For this review, use the dimensioned drawing (mm, ordinates from the lowest corner) and the shaded views. Coordinates: 2 decimals unless noted, no trailing zeros. Loops run counter-clockwise (first coordinate to the right, second up) from the corner with the lowest first, then second, coordinate; pieces in that order, holes last. Notation, with made-up numbers: (27, 19.5) -> (70, 19.5) arc R25 cw to (70, 31.5) -> close; hole circle Ø9 at (-3.5, 71). An arc over 180 degrees is marked (long way). Answer as a JSON object with one key per item and string values.
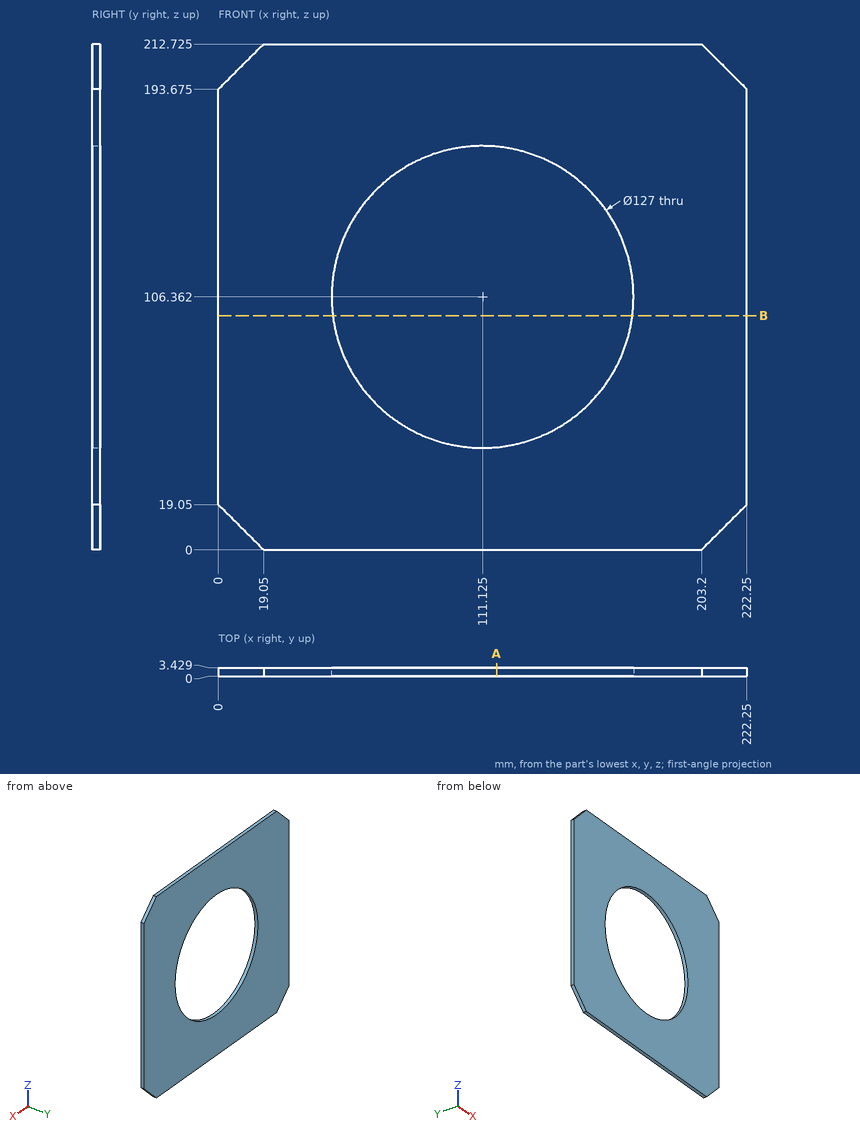
1) Add section A-A, the plane x = 117. Give the boundary of the cut face in (y, z) (1 decimal), and give its area (3 significant figures).
Completed:
{"outline": "(0, 0) -> (3.4, 0) -> (3.4, 43.1) -> (0, 43.1) -> close; (0, 169.6) -> (3.4, 169.6) -> (3.4, 212.7) -> (0, 212.7) -> close", "area": "296 mm²"}
2) Add section B-B, the plane z = 98.5. Give the boundary of the cut face in (x, y).
Completed:
{"outline": "(0, 0) -> (48.11, 0) -> (48.11, 3.43) -> (0, 3.43) -> close; (174.14, 0) -> (222.25, 0) -> (222.25, 3.43) -> (174.14, 3.43) -> close"}
3) Wall thickness on probe 1 along Z at (x, y) = (66.5, 1.75) (1 decimal); probe 2 along Z at (x, y) = (78, 1.05) (1 decimal); probe 3 along X at (y, z) = (1.7, 122.5): over which ranges is each line inside the solid? List them lowest first.
Completed:
{"probe 1": "0 to 61.2, 151.5 to 212.7", "probe 2": "0 to 52.2, 160.5 to 212.7", "probe 3": "0 to 49.71, 172.54 to 222.25"}
